CAD build for the part. Positions are in the model's coordinates, mm. Face numbers are marked on the shaded views. A direction names the side the tool comes from. Coordinates: 2 decimals unless noted, no trailing zeros. Order: outer loops, then holes, each group sorted by start corner. A loop starts at its lowest first (then second) coordinate and runs counter-clockwise, first axis right, second up. Notation, with made-up numbers: (41.25, 40) - (91.25, 40) arc R33 cw to (91.25, 74) - close; hole circle Ø5 at (24, -5). An arc over 180 degrees is marked (long way). Return JSON: item names as keys, results as strings.
from build123d import *

# Parameters (mm, degrees)
F0_W      = 125
F0_H      = 70
F1_DEPTH  = 15
F3_DEPTH  = 70
F5_DEPTH  = 70
F7_DEPTH  = 70
F9_DEPTH  = 20
F11_DEPTH = 20
F12_W     = 15
F12_H     = 30
F13_DEPTH = 72


with BuildPart() as f1:
    # F0 (on Top) → F1 (new body)
    with BuildSketch(Plane.XY):
        Rectangle(F0_W, F0_H)
    extrude(amount=F1_DEPTH)

    # F2 (on face) → F3 (join)
    with BuildSketch(Plane.XZ.offset(35)):
        Polygon((62.5, 15), (62.5, 0), (72.5, 0), align=None)
    extrude(amount=-F3_DEPTH)

    # F4 (on face) → F5 (join)
    with BuildSketch(Plane.XZ.offset(35)):
        Polygon((-77.5, 0), (-62.5, 0), (-62.5, 15), align=None)
    extrude(amount=-F5_DEPTH)

    # F6 (on face) → F7 (join)
    with BuildSketch(Plane(origin=(0, 35, 0), x_dir=(-1, 0, 0), z_dir=(0, 1, 0))):
        Polygon((-17.0299803775, 83.2050294338), (-62.5, 15), (-47.5, 15), (-2.0299803775, 83.2050294338), align=None)
    extrude(amount=-F7_DEPTH)

    # F8 (on face) → F9 (join)
    with BuildSketch(Plane.XZ.offset(35)):
        with BuildLine():
            Line((2.0299803775, 163.2050294338), (2.0299803775, 83.2050294338))
            Line((2.0299803775, 83.2050294338), (17.0299803775, 83.2050294338))
            Line((17.0299803775, 83.2050294338), (17.0299803775, 163.2050294338))
            ThreePointArc((17.0299803775, 163.2050294338), (9.5299803775, 155.7050294338), (2.0299803775, 163.2050294338))
        make_face()
        with BuildLine():
            ThreePointArc((17.0299803775, 163.2050294338), (9.5299803775, 170.7050294338), (2.0299803775, 163.2050294338))
            Line((2.0299803775, 163.2050294338), (5.5299803775, 163.2050294338))
            ThreePointArc((5.5299803775, 163.2050294338), (9.5299803775, 167.2050294338), (13.5299803775, 163.2050294338))
            Line((13.5299803775, 163.2050294338), (17.0299803775, 163.2050294338))
        make_face()
        with BuildLine():
            Line((5.5299803775, 163.2050294338), (2.0299803775, 163.2050294338))
            ThreePointArc((2.0299803775, 163.2050294338), (9.5299803775, 155.7050294338), (17.0299803775, 163.2050294338))
            Line((17.0299803775, 163.2050294338), (13.5299803775, 163.2050294338))
            ThreePointArc((13.5299803775, 163.2050294338), (9.5299803775, 159.2050294338), (5.5299803775, 163.2050294338))
        make_face()
    extrude(amount=-F9_DEPTH)

    # F10 (on face) → F11 (join)
    with BuildSketch(Plane(origin=(0, 35, 0), x_dir=(-1, 0, 0), z_dir=(0, 1, 0))):
        with BuildLine():
            Line((-17.0299803775, 163.2050294338), (-17.0299803775, 83.2050294338))
            Line((-17.0299803775, 83.2050294338), (-2.0299803775, 83.2050294338))
            Line((-2.0299803775, 83.2050294338), (-2.0299803775, 163.2050294338))
            ThreePointArc((-2.0299803775, 163.2050294338), (-9.5299803775, 155.7050294338), (-17.0299803775, 163.2050294338))
        make_face()
        with BuildLine():
            ThreePointArc((-2.0299803775, 163.2050294338), (-9.5299803775, 170.7050294338), (-17.0299803775, 163.2050294338))
            Line((-17.0299803775, 163.2050294338), (-13.5299803775, 163.2050294338))
            ThreePointArc((-13.5299803775, 163.2050294338), (-9.5299803775, 167.2050294338), (-5.5299803775, 163.2050294338))
            Line((-5.5299803775, 163.2050294338), (-2.0299803775, 163.2050294338))
        make_face()
        with BuildLine():
            Line((-13.5299803775, 163.2050294338), (-17.0299803775, 163.2050294338))
            ThreePointArc((-17.0299803775, 163.2050294338), (-9.5299803775, 155.7050294338), (-2.0299803775, 163.2050294338))
            Line((-2.0299803775, 163.2050294338), (-5.5299803775, 163.2050294338))
            ThreePointArc((-5.5299803775, 163.2050294338), (-9.5299803775, 159.2050294338), (-13.5299803775, 163.2050294338))
        make_face()
    extrude(amount=-F11_DEPTH)

    # F12 (on face) → F13 (join)
    with BuildSketch(Plane.XY.offset(83.2050294338)):
        with Locations((9.5299803775, 0)):
            Rectangle(F12_W, F12_H)
    extrude(amount=F13_DEPTH)


solid = f1.part
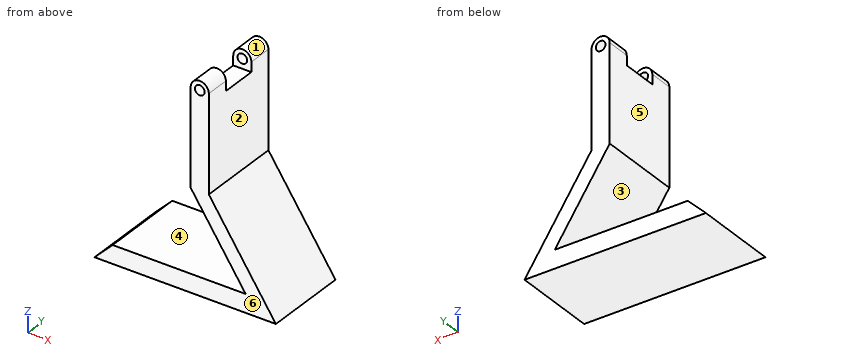
Item 1: Band-saw the part on D-D, the plane z = 142. List the corners of the cut face in (x, y).
Findings below:
{"outline": "(2.03, -35) - (17.03, -35) - (17.03, 35) - (2.03, 35) - close"}
Item 2: Drop flat-ended pins along their axis: P1, Ø5, axis at y = 4, z = 102.5, coming from the -X side; P2, Ø7, axis at x = 9.53, z = 163.21, coming from the -Y side; P3, Ø10, axis at y = 9, z = 147.5, coming from the +X side; P4, Ø6, axis at y = -0.5, z = 18.5, coming from the +X side. Give the stop position or say it passes through.
Findings below:
{"P1": "stops at x = 2.03", "P2": "passes through", "P3": "stops at x = 17.03", "P4": "stops at x = 62.17"}
Item 3: Band-saw the part on B-B, the plane y = -17. List the corners of the cut face in (x, z), then the cut area to 3 significant figures.
Findings below:
{"outline": "(-77.5, 0) - (72.5, 0) - (17.03, 83.21) - (17.03, 163.21) arc R7.5 ccw to (2.03, 163.21) - (2.03, 83.21) - (47.5, 15) - (-62.5, 15) - close; hole circle Ø8 at (9.53, 163.21)", "area": "4,320 mm²"}
Item 4: Which spindle directions (+Z, -Z, +X, -X, +Y, -Y) get a long thin tool onto all of the face, cutting with end or side? Do the marked faces 4, 5 and 6. Say none if no direction does.
Findings below:
{"face 4": "-X, +Y, -Y", "face 5": "+Z, -X, +Y, -Y", "face 6": "+Z, -Z, +X, -X, -Y"}
Item 5: Wall check: L1, parallel to Z at x = -28, y = -11; L2, parallel to X at y = 15, z = 121; L3, parallel to Z at x = 13, y = -6.5. Give the ranges that are in metal, low to high. Write a range as [from, to].
Findings below:
{"L1": "z = [0, 15]", "L2": "x = [2.03, 17.03]", "L3": "z = [0, 15], [66.75, 155.21]"}
Item 6: Band-saw the part on A-A, the plane x = 27.5. List the corners of the cut face in (y, z), then the cut area to 4 significant figures.
Findings below:
{"outline": "(-35, 0) - (35, 0) - (35, 15) - (-35, 15) - close; (-35, 45) - (35, 45) - (35, 67.5) - (-35, 67.5) - close", "area": "2,625 mm²"}
Item 7: Mould opens along Z. For the marked faces 1, 2 and 3 say: released by +Z, released by -Z, zero draft, split by the parting line, or undercut.
Findings below:
{"face 1": "released by +Z", "face 2": "zero draft", "face 3": "undercut"}
Item 8: Band-saw the part on C-C, the plane y = -3.5. List the corners of the cut face in (x, z).
Findings below:
{"outline": "(-77.5, 0) - (72.5, 0) - (17.03, 83.21) - (17.03, 155.21) - (2.03, 155.21) - (2.03, 83.21) - (47.5, 15) - (-62.5, 15) - close"}
